Verification items for the finished model (mm, model axes). Face numbers are marked on the shaded views. Give positions to 0.01 mm unless a question says otherwise; leave off trailing zeros. Loops run counter-clockwise (first coordinate to the right, second up) from the corner with the lowest first, then second, coordinate; pieces in that order, holes last. Notation, with made-up numbers: (-25.5, -27) - (4.5, -27) arc R21 ccw to (4.5, -13) - close; hole circle Ø1 at (65.5, -22.75). An arc over 180 degrees is marked (long way). Answer in a Markdown table with one row per item.
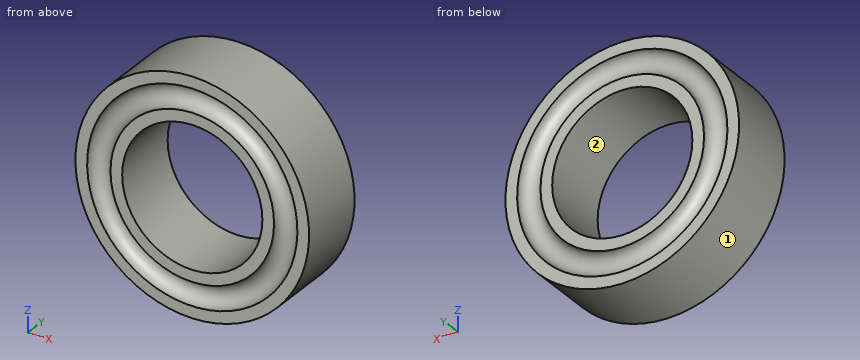
```python
from build123d import *

# Parameters (mm, degrees)
SKETCH2_R          = 3
CUT_EXTRUDE1_DEPTH = 10


with BuildPart() as part:
    # Sketch1 → Revolve1 (revolve)
    with BuildSketch(Plane.XY, mode=Mode.PRIVATE) as revolve1_sk:
        with BuildLine():
            Line((0, 1.5), (3.5, 1.5))
            ThreePointArc((3.5, 1.5), (4, 1), (4.5, 1.5))
            Line((4.5, 1.5), (5, 1.5))
            Line((5, 1.5), (5, -1.5))
            Line((5, -1.5), (4.5, -1.5))
            ThreePointArc((4.5, -1.5), (4, -1), (3.5, -1.5))
            Line((3.5, -1.5), (0, -1.5))
            Line((0, -1.5), (0, 1.5))
        make_face()
    revolve(revolve1_sk.sketch.rotate(Axis((0, 2.010416667, 0), (0, -1, 0)), 90), axis=Axis((0, 2.010416667, 0), (0, -1, 0)))

    # Sketch2 → Cut-Extrude1 (cut)
    with BuildSketch(Plane(origin=(0, 1.5, 0), x_dir=(1, 0, 0), z_dir=(0, 1, 0))):
        with Locations(Location((0, 0, 0), (0, 0, 270))):
            Circle(SKETCH2_R)
    extrude(amount=-CUT_EXTRUDE1_DEPTH, mode=Mode.SUBTRACT)


solid = part.part
```
Q1. Sectioned sample at B-B (x = 0). Record the cut outline in (y, z).
Completed:
| item | result |
|---|---|
| outline | (-1.5, -5) - (1.5, -5) - (1.5, -4.5) arc R0.5 cw to (1.5, -3.5) - (1.5, -3) - (-1.5, -3) - (-1.5, -3.5) arc R0.5 cw to (-1.5, -4.5) - close; (-1.5, 3) - (1.5, 3) - (1.5, 3.5) arc R0.5 cw to (1.5, 4.5) - (1.5, 5) - (-1.5, 5) - (-1.5, 4.5) arc R0.5 cw to (-1.5, 3.5) - close |
Q2. Sectioned sample at C-C (y = -1.2). Record the cut outline in (x, z), and give its area (3 significant figures).
Completed:
| item | result |
|---|---|
| outline | circle Ø10 at (0, 0); circle Ø7.2 at (0, 0); hole circle Ø8.8 at (0, 0); hole circle Ø6 at (0, 0) |
| area | 30.2 mm^2 |
Q3. Sectioned sample at D-D (y = 0.25). Record the cut outline in (x, z).
Completed:
| item | result |
|---|---|
| outline | circle Ø10 at (0, 0); hole circle Ø6 at (0, 0) |
Q4. Thickness scan on line 1 (X direction, y = 0, z = 0); line 2 (X direction, y = 1.35, z = -1); line 3 (Z direction, x = -2, y = -1.1). Record the ranges inside material, lowest first.
Completed:
| item | result |
|---|---|
| line 1 | -5 to -3, 3 to 5 |
| line 2 | -4.9 to -4.36, -3.38 to -2.83, 2.83 to 3.38, 4.36 to 4.9 |
| line 3 | -4.58 to -3.81, -3.11 to -2.24, 2.24 to 3.11, 3.81 to 4.58 |
Q5. Sectioned sample at A-A (z = 0). Record the cut outline in (x, y).
Completed:
| item | result |
|---|---|
| outline | (-5, -1.5) - (-4.5, -1.5) arc R0.5 cw to (-3.5, -1.5) - (-3, -1.5) - (-3, 1.5) - (-3.5, 1.5) arc R0.5 cw to (-4.5, 1.5) - (-5, 1.5) - close; (3, -1.5) - (3.5, -1.5) arc R0.5 cw to (4.5, -1.5) - (5, -1.5) - (5, 1.5) - (4.5, 1.5) arc R0.5 cw to (3.5, 1.5) - (3, 1.5) - close |
Q6. Go/stop test with flat-tipped pins: P1, Ø1.5, axis at x = 2.5, y = 0.5, coming from the -Z side; P2, Ø1.5, axis at x = 4, y = -0.5, coming from the -Z side. Record where each tip stops, or that it passes through.
Completed:
| item | result |
|---|---|
| P1 | z = -4.68 |
| P2 | z = -3.8 |
Q7. Draft check along X on the marked faces 1 and 2. Enter one of: +X half, -X half, draft (parallel to the pull), parting line (faces both ways), or undercut.
Completed:
| item | result |
|---|---|
| face 1 | parting line |
| face 2 | undercut |
